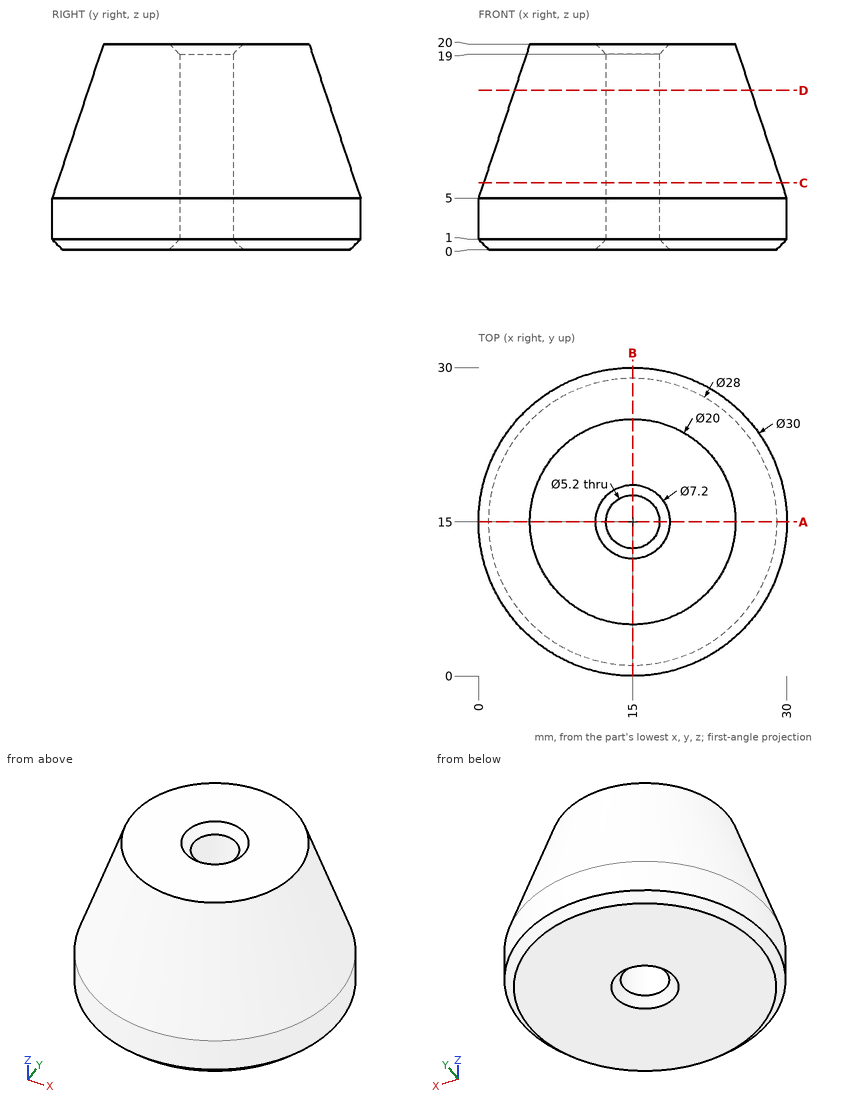
Could you check a few things on this drawing? It's one solid part, dimensions in mm from its lowest x, y, z. Coordinates: 2 decimals unless noted, no trailing zeros. Loops run counter-clockwise (first coordinate to the right, second up) from the corner with the lowest first, then second, coordinate; pieces in that order, holes last. Notation, with made-up numbers: (81.5, -2.5) - (116.5, -2.5) arc R10 ccw to (116.5, 1.5) - close; hole circle Ø11 at (-17, 83.25). An arc over 180 degrees is marked (long way). Return JSON: item names as keys, results as strings. Group by question number.
Item 1: If we section it at C-C on z = 6.5: Write out the boundary of the cut face in (x, y), and give its area (3 significant figures).
Item 2: If we section it at D-D on z = 15.5: Write out the boundary of the cut face in (x, y).
Item 3: Will these pins go through, and if not, where does the flat tip stop? P1, Ø1.5, axis at x = 26, z = 13, coming from the +Y side; P2, Ø2, axis at y = 10, z = 13, coming from the +X side; P3, Ø6, axis at x = 15, y = 15, coming from the +Z side.
Item 4: I need wall thicknesses on line 1 (Y direction, x = 17.25, z = 16.5); line 2 (Y direction, x = 15, z = 15.75); line 3 (X direction, y = 15, z = 8.75). Which ranges of each line are inside material? Lowest first, please. Write a range as from..to.
Item 5: If we section it at A-A on y = 15: Write out the boundary of the cut face in (x, z).
Calculated:
{
 "1": {"outline": "circle Ø29 at (15, 15); hole circle Ø5.2 at (15, 15)", "area": "639 mm^2"},
 "2": {"outline": "circle Ø23 at (15, 15); hole circle Ø5.2 at (15, 15)"},
 "3": {"P1": "stops at y = 21.95", "P2": "stops at x = 26.81", "P3": "stops at z = 19.4"},
 "4": {"line 1": "y = 4.06..13.7, 16.3..25.94", "line 2": "y = 3.58..12.4, 17.6..26.42", "line 3": "x = 1.25..12.4, 17.6..28.75"},
 "5": {"outline": "(0, 1) - (1, 0) - (11.4, 0) - (12.4, 1) - (12.4, 19) - (11.4, 20) - (5, 20) - (0, 5) - close; (17.6, 1) - (18.6, 0) - (29, 0) - (30, 1) - (30, 5) - (25, 20) - (18.6, 20) - (17.6, 19) - close"}
}
